Check sheet for the modelled part. Datum: model origin and axes. Units: mm. A direction names the side the tool comes from. Coordinates: 2 decimals unless noted, no trailing zeros. Write each loop counter-clockwise with the first axis right and the second up, starting at its lowest first coordinate (ties: lowest second). Pieces come first, ordered by that corner, then holes. Notation, with made-up numbers: (-23, 41) - (17, 41) arc R29 ccw to (17, 76) - close; hole circle Ø11 at (-38.5, -30.5). An arc over 180 degrees is marked (long way). Write each question's results on one line, items separated by ' | '.
from build123d import *

# Parameters (mm, degrees)
F0_W     = 1500
F0_H     = 1200
F1_DEPTH = 200
F2_R     = 5
F3_W     = 1350
F3_H     = 895
F4_DEPTH = 80
F5_R     = 40
F6_W     = 1400
F6_H     = 945
F6_W_2   = 1350
F6_H_2   = 895
F7_DEPTH = 70


with BuildPart() as f1:
    # F0 (on Front) → F1 (new body)
    with BuildSketch(Plane.XZ):
        with Locations((-750, 600)):
            Rectangle(F0_W, F0_H)
    extrude(amount=F1_DEPTH)

    # F2
    f2_edges = [f1.edges().sort_by_distance(p)[0] for p in [
        (-1500, -100, 1200),
        (0, -100, 1200),
        (-750, 0, 1200),
        (-750, -200, 1200),
        (-1500, -200, 600),
        (-1500, 0, 600),
        (0, -200, 600),
        (0, 0, 600),
    ]]
    fillet(f2_edges, radius=F2_R)

    # F3 (on face) → F4 (cut)
    with BuildSketch(Plane.XZ.offset(200)):
        with Locations((-750, 627.5)):
            Rectangle(F3_W, F3_H)
    extrude(amount=-F4_DEPTH, mode=Mode.SUBTRACT)

    # F5
    f5_edges = [f1.edges().sort_by_distance(p)[0] for p in [
        (-750, -120, 180),
        (-750, -120, 1075),
    ]]
    fillet(f5_edges, radius=F5_R)

    # F6 (on face) → F7 (cut)
    with BuildSketch(Plane.XZ.offset(200)):
        with Locations((-750, 627.5)):
            Rectangle(F6_W, F6_H)
        with Locations((-750, 627.5)):
            Rectangle(F6_W_2, F6_H_2, mode=Mode.SUBTRACT)
    extrude(amount=-F7_DEPTH, mode=Mode.SUBTRACT)


solid = f1.part
1. Access from +Z, -Z, +X, -X, +Y, -Y to the whole of each face (thin tool, end or side, straight path). Record for faces 4 (the flat face through (-760, -99, 1200)), 5 (the flat face through (-759, -145, 180)).
Values follow:
face 4: +Z, +X, -X, +Y, -Y | face 5: -Y
2. Draft check along X on faces 1 (the cylindrical face through (-740.55, -132.028, 1063.594)), 2 (the flat face through (-760, -99, 0)), 3 (the flat face through (-1500, -99, 589)). Enter one of: pulls with the +X half, pulls with the -X half, needs draft (parallel to the pull), parting line crosses it, or undercut.
Values follow:
face 1: undercut | face 2: needs draft | face 3: pulls with the -X half
3. Sectioned sample at B-B (x = -1054). Record the cut outline in (y, z).
Values follow:
outline: (-200, 0) - (0, 0) - (0, 1195) arc R5 ccw to (-5, 1200) - (-195, 1200) arc R5 ccw to (-200, 1195) - (-200, 1100) - (-130, 1100) - (-130, 1075) - (-160, 1075) arc R40 cw to (-120, 1035) - (-120, 220) arc R40 cw to (-160, 180) - (-130, 180) - (-130, 155) - (-200, 155) - close
4. Material ranges on L1, parallel to X at y = -188.5, z = 455; L2, parallel to Z at x = -191, y = -153; L3, parallel to Y at x = -221.5, z = 229, recorded low to high. Write a range as [from, to].
Values follow:
L1: x = [-1500, -1450], [-50, 0] | L2: z = [0, 155], [180, 180.62], [1074.38, 1075], [1100, 1200] | L3: y = [-120, 0]
5. Sectioned sample at A-A (z = 564). Record the cut outline in (x, y), then the cut area to 3 significant figures.
Values follow:
outline: (-1500, -195) arc R5 ccw to (-1495, -200) - (-1450, -200) - (-1450, -130) - (-1425, -130) - (-1425, -120) - (-75, -120) - (-75, -130) - (-50, -130) - (-50, -200) - (-5, -200) arc R5 ccw to (0, -195) - (0, -5) arc R5 ccw to (-5, 0) - (-1495, 0) arc R5 ccw to (-1500, -5) - close | area: 188,000 mm^2
